Geometry: final body of the model. Coordinates: model frame, mm. A direction names the side the tool comes from. Give positions to 0.01 mm unless a question says otherwise; leave off trailing zeros. Write each loop counter-clockwise with the first axis right and the second up, starting at its lowest first coordinate (ties: lowest second). Pieces come first, ordered by that corner, then holes.
Q1. Line query: L1, parallel to X at y = 19.5, z = 3; L2, parallel to Z at x = -13, y = 5; L3, parallel to Y at x = -15, z = 11.5. Output: solid intervals per line, ascending.
Q2. Reachability of faces 1 (the face through (20.274, -14.924, 5.241)), 2 (the face through (0, 15, 15)), 3 (the face through (0, 0, 0)) from +Z, -Z, +X, -X, +Y, -Y: full face, straight path, thin tool, end or side. Return the list, or none.
Q3. Cut plane B-B on x = 0. Return the cut outline in (y, z), plus the area to 3 significant figures.
Q4. Cut plane A-A on y = 28.5. Return the cut outline in (x, z).
Q5. Pin query (flat end, axial travel): pin 1 (11.5 mm diameter, centred on y = -20, z = 15, fed in from +X); pin 2 (10 mm diameter, centred on x = -1, z = 11.5, fed in from +Y). Return the tip coordinate at first contact, or that it passes through.
Q6. Cut plane D-D on y = -20. Return the cut outline in (x, z), plus the area to 3 significant figures.
Q7. Draft query along Y for faces 4 (the face through (-16, 35, 15)), 5 (the face through (2.307, -24.436, 24.456)), 6 (the face through (-10, 25, 15)), 7 (the face through (18.5, -15, 13)). Return one class per face: pulls with the +Y half, pulls with the -Y half, needs draft (parallel to the pull), parting line crosses it, or undercut.
Q8. Cut plane C-C on z = 15. Return the cut outline in (x, y).
```python
from build123d import *

# Parameters (mm, degrees)
CROQUIS1_R              = 5
SALIENTE_EXTRUIR1_DEPTH = 30
CROQUIS2_R              = 11
CORTAR_EXTRUIR1_DEPTH   = 3.5
CROQUIS3_R              = 5.1
CORTAR_EXTRUIR2_DEPTH   = 62.361632964
CROQUIS4_R              = 4
CORTAR_EXTRUIR3_DEPTH   = 64.725975982


with BuildPart() as part:
    # Croquis1 → Saliente-Extruir1 (new body)
    with BuildSketch(Plane.XY):
        Polygon((-10, 35), (-22, 35), (-22, -35), (22, -35), (22, 35), (10, 35), (10, 15), (-10, 15), align=None)
        with Locations((0, -20)):
            Circle(CROQUIS1_R, mode=Mode.SUBTRACT)
    extrude(amount=SALIENTE_EXTRUIR1_DEPTH)

    # Croquis2 → Cortar-Extruir1 (cut)
    with BuildSketch(Plane(origin=(22, 0, 0), x_dir=(0, 0, -1), z_dir=(1, 0, 0))):
        with Locations(Location((-15, -20, 0), (0, 0, 90))):
            Circle(CROQUIS2_R)
    extrude(amount=-CORTAR_EXTRUIR1_DEPTH, mode=Mode.SUBTRACT)

    # Croquis3 → Cortar-Extruir2 (cut, through all)
    with BuildSketch(Plane(origin=(18.5, 0, 0), x_dir=(0, 0, -1), z_dir=(1, 0, 0))):
        with Locations(Location((-15, -20, 0), (0, 0, 90))):
            Circle(CROQUIS3_R)
    extrude(amount=-CORTAR_EXTRUIR2_DEPTH, mode=Mode.SUBTRACT)

    # Croquis4 → Cortar-Extruir3 (cut, through all)
    with BuildSketch(Plane(origin=(22, 0, 0), x_dir=(0, 0, -1), z_dir=(1, 0, 0))):
        with Locations(Location((-15, 5, 0), (0, 0, 90))):
            Circle(CROQUIS4_R)
    extrude(amount=-CORTAR_EXTRUIR3_DEPTH, mode=Mode.SUBTRACT)


solid = part.part
```
Data:
1. L1: x = -22 to -10, 10 to 22
1. L2: z = 0 to 11, 19 to 30
1. L3: y = -35 to -23.71, -16.29 to 3.06, 6.94 to 35
2. face 1: +X
2. face 2: +Z, -Z, +Y
2. face 3: -Z, +X, -X, +Y, -Y
3. outline: (-35, 0) - (-25, 0) - (-25, 14) arc R5.1 cw to (-25, 16) - (-25, 30) - (-35, 30) - close; (-15, 0) - (15, 0) - (15, 30) - (-15, 30) - (-15, 16) arc R5.1 cw to (-15, 14) - close; hole circle Ø8 at (5, 15)
3. area: 1,150 mm2
4. outline: (-22, 0) - (-10, 0) - (-10, 30) - (-22, 30) - close; (10, 0) - (22, 0) - (22, 30) - (10, 30) - close
5. pin 1: stops at x = 18.5
5. pin 2: stops at y = 15
6. outline: (-22, 0) - (-5, 0) - (-5, 9.9) - (-22, 9.9) - close; (-22, 20.1) - (-5, 20.1) - (-5, 30) - (-22, 30) - close; (5, 0) - (22, 0) - (22, 4) - (18.5, 4) - (18.5, 9.9) - (5, 9.9) - close; (5, 20.1) - (18.5, 20.1) - (18.5, 26) - (22, 26) - (22, 30) - (5, 30) - close
6. area: 632 mm2
7. face 4: pulls with the +Y half
7. face 5: undercut
7. face 6: needs draft
7. face 7: undercut
8. outline: (-22, -35) - (22, -35) - (22, -31) - (18.5, -31) - (18.5, -25.1) - (-22, -25.1) - close; (-22, -14.9) - (18.5, -14.9) - (18.5, -9) - (22, -9) - (22, 1) - (-22, 1) - close; (-22, 9) - (22, 9) - (22, 35) - (10, 35) - (10, 15) - (-10, 15) - (-10, 35) - (-22, 35) - close
